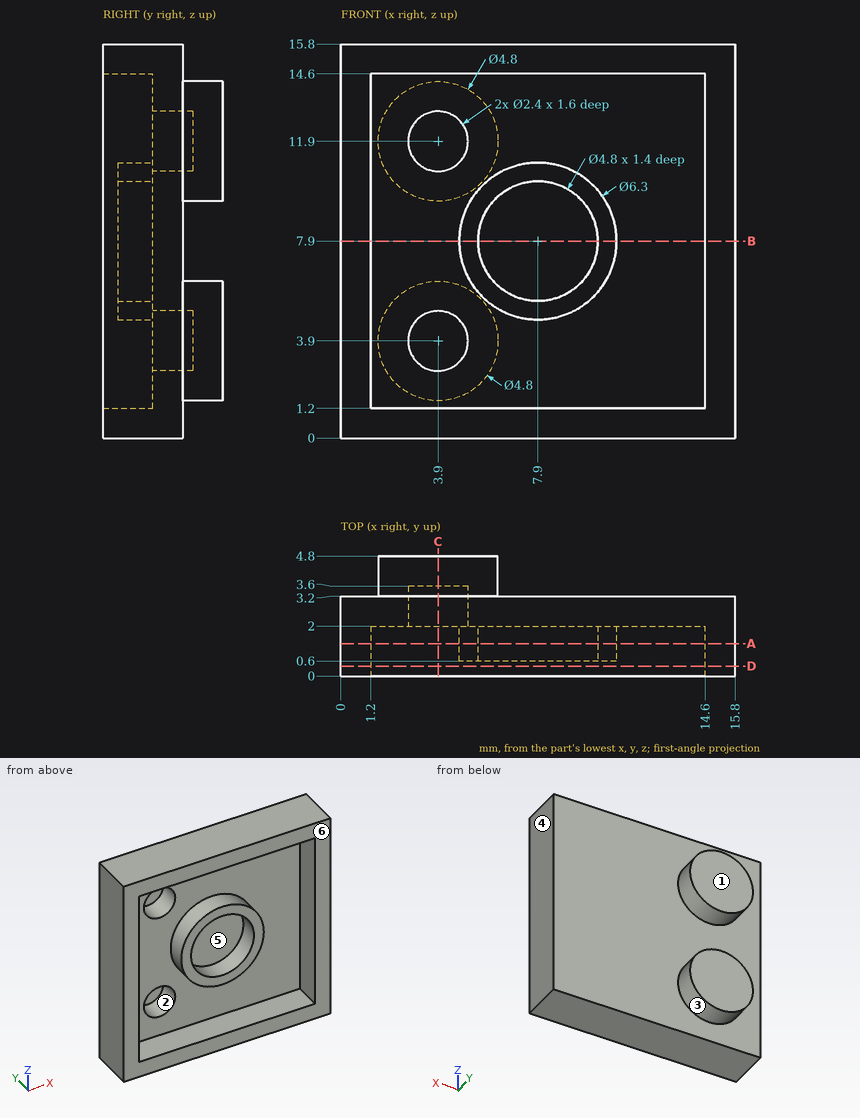
For this review, use the dimensioned drawing (mm, ordinates from the lowest corner) and the shaded views. A direction names the side the tool comes from. Give positions to 0.01 mm unless a question says otherwise; leave off trailing zeros. Order: outer loops, then holes, each group sorted by start corner. A loop starts at its lowest first (then second) coordinate and runs counter-clockwise, first axis right, second up.
1) Take a section at A-A (y = 1.3). Give the boundary of the cut face in (x, z).
2) Take a section at B-B (z = 7.9). Give the boundary of the cut face in (x, y), then the cut area to 3 significant figures.
3) Wall thickness on line 1 (Z direction, x = 7.9, y = 1.05); line 2 (Z direction, x = 3.9, y = 2.95): over which ranges is each line inside the solid? List them lowest first.
4) The part is to be moulded in two halves that separate along X. For the marked faces 4, 5 and 6, say which applies: released by +X, released by -X, zero draft, split by the parting line, or undercut.
5) For the marked faces 1, 2 and 3, list the 3-axis set-ups (+Z, -Z, +X, -X, +Y, -Y) from which the entire face can be reached by the end or side of a thin tool; tool diameter is ignored.
6) Take a section at D-D (y = 0.4). Give the boundary of the cut face in (x, z).
7) Insertion check: pin 1 (1 mm diameter, centred on y = 2.5, z = 12, fed in from -X); pin 2 (2.5 mm diameter, centred on x = 4, z = 11.5, fed in from -Y); pin 3 (5.5 mm diameter, centred on x = 7.5, z = 7, fed in from -Y); pin 4 (4 mm diameter, centred on x = 11, z = 12, fed in from +Y). Each pin has a flat end and moves straight along its axis. Give the tip position at first contact, or say it passes through.
8) Take a section at C-C (x = 3.9). Give the boundary of the cut face in (y, z).
Derived:
1. outline: (0, 0) - (15.8, 0) - (15.8, 15.8) - (0, 15.8) - close; circle Ø6.3 at (7.9, 7.9); hole (1.2, 1.2) - (14.6, 1.2) - (14.6, 14.6) - (1.2, 14.6) - close; hole circle Ø4.8 at (7.9, 7.9)
2. outline: (0, 0) - (1.2, 0) - (1.2, 2) - (4.75, 2) - (4.75, 0.6) - (5.5, 0.6) - (5.5, 2) - (10.3, 2) - (10.3, 0.6) - (11.05, 0.6) - (11.05, 2) - (14.6, 2) - (14.6, 0) - (15.8, 0) - (15.8, 3.2) - (0, 3.2) - close
2. area: 25.9 mm2
3. line 1: z = 0 to 1.2, 4.75 to 5.5, 10.3 to 11.05, 14.6 to 15.8
3. line 2: z = 0 to 2.7, 5.1 to 10.7, 13.1 to 15.8
4. face 4: released by +X
4. face 5: undercut
4. face 6: zero draft
5. face 1: +Z, -Z, +X, -X, +Y
5. face 2: -Y
5. face 3: +Y
6. outline: (0, 0) - (15.8, 0) - (15.8, 15.8) - (0, 15.8) - close; hole (1.2, 1.2) - (14.6, 1.2) - (14.6, 14.6) - (1.2, 14.6) - close
7. pin 1: stops at x = 0
7. pin 2: stops at y = 2
7. pin 3: stops at y = 0.6
7. pin 4: stops at y = 3.2
8. outline: (0, 0) - (3.2, 0) - (3.2, 1.5) - (4.8, 1.5) - (4.8, 6.3) - (3.2, 6.3) - (3.2, 9.5) - (4.8, 9.5) - (4.8, 14.3) - (3.2, 14.3) - (3.2, 15.8) - (0, 15.8) - (0, 14.6) - (2, 14.6) - (2, 13.1) - (3.6, 13.1) - (3.6, 10.7) - (2, 10.7) - (2, 5.1) - (3.6, 5.1) - (3.6, 2.7) - (2, 2.7) - (2, 1.2) - (0, 1.2) - close
